Geometry: see drawing. Coordinates: mm, zero at the bounding-box minimum. Coordinates: 2 decimals unless noted, no trailing zeros. Loops run counter-clockwise (first coordinate to the right, second up) from the corner with the lowest first, then second, coordinate; pieces in that order, holes last. Notation, with made-up numbers: (22, 74.25) -> (81, 74.25) arc R23 ccw to (81, 83.25) -> close; hole circle Ø8 at (35.25, -30). An arc over 180 degrees is marked (long way). Put each result on its own line as item: value. Start each with the question number.
1) Cut plane D-D (x = 28). Return the cut outline in (y, z) (1 decimal), plus the area to 3 significant figures.
2) Cut plane C-C (y = 42.5). Return the cut outline in (x, z).
3) Cut plane B-B (z = 1.4). Return the cut outline in (x, y).
4) Material intervals for L1, parallel to Y at x = 65, z = 1.7; L2, parallel to X at y = 18, z = 0.45; L3, parallel to Y at x = 57.5, z = 1, sorted ascending.
5) Cut plane A-A (x = 65). Return the cut outline in (y, z).
6) Contact query for flat-ended pins moving along their axis: P1, Ø3, axis at y = 57.5, z = 3.5, coming from the -X side; P2, Ø2, axis at y = 42.5, z = 2.5, coming from the +X side; P3, Ø1, axis at y = 23, z = 3, coming from the -X side (1 decimal). Output: stop coordinate, or through.
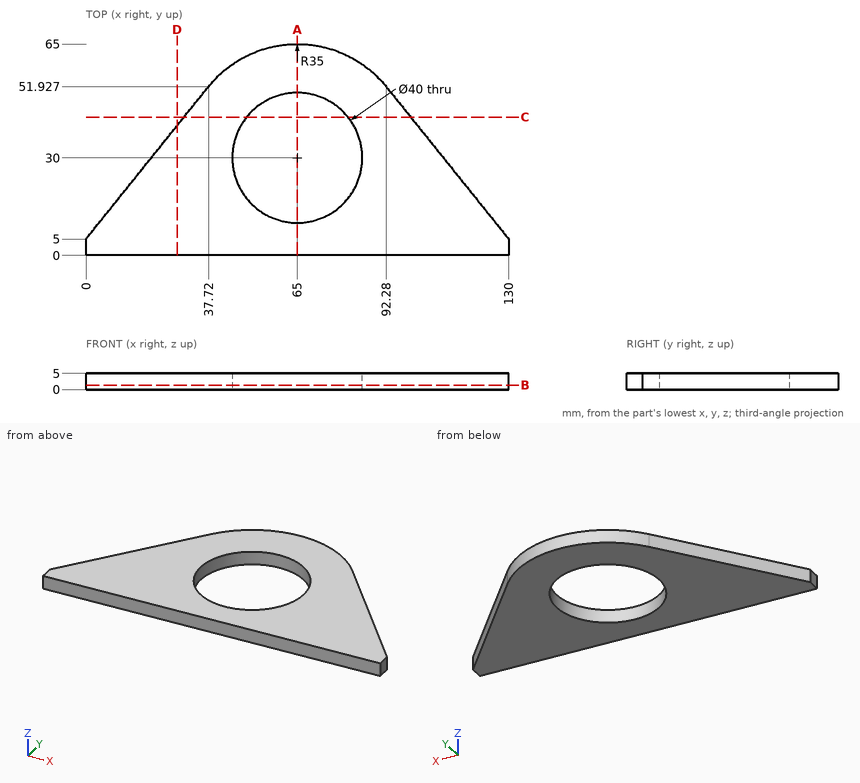
Results found:
1. outline: (0, 0) -> (39.8, 0) -> (39.8, 5) -> (0, 5) -> close
1. area: 199 mm2
2. outline: (30.14, 0) -> (49.39, 0) -> (49.39, 5) -> (30.14, 5) -> close; (80.61, 0) -> (99.86, 0) -> (99.86, 5) -> (80.61, 5) -> close
3. outline: (0, 0) -> (130, 0) -> (130, 5) -> (92.28, 51.93) arc R35 ccw to (37.72, 51.93) -> (0, 5) -> close; hole circle Ø40 at (65, 30)
4. L1: y = 0 to 10, 50 to 65
4. L2: x = 10.45 to 49, 81 to 119.55
4. L3: y = 0 to 11.46, 48.54 to 64.19
5. outline: (0, 0) -> (10, 0) -> (10, 5) -> (0, 5) -> close; (50, 0) -> (65, 0) -> (65, 5) -> (50, 5) -> close
6. P1: stops at x = 41.57
6. P2: stops at x = 100.66
6. P3: stops at x = 14.1
